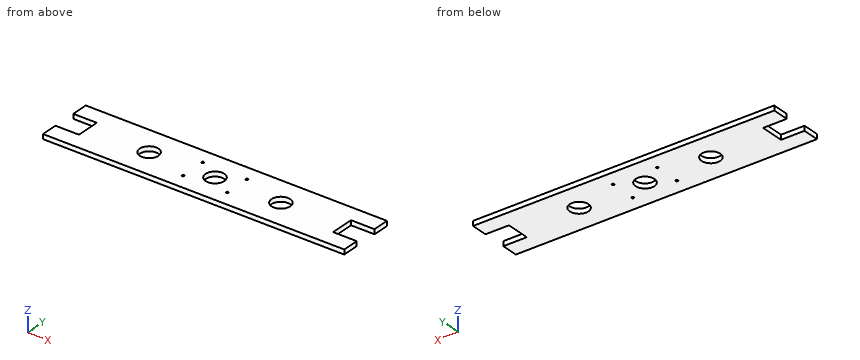
from build123d import *

# Parameters (mm, degrees)
F0_R     = 3.175
F0_R_2   = 25.4
F1_DEPTH = 12.7


with BuildPart() as f1:
    # F0 (on Top) → F1 (new body)
    with BuildSketch(Plane.XY):
        Polygon((406.4, 76.2), (-406.4, 76.2), (-406.4, 31.75), (-342.9, 31.75), (-342.9, -31.75), (-406.4, -31.75), (-406.4, -76.2), (406.4, -76.2), (406.4, -31.75), (342.9, -31.75), (342.9, 31.75), (406.4, 31.75), align=None)
        with Locations((-59.5122, -34.925)):
            Circle(F0_R, mode=Mode.SUBTRACT)
        with Locations((59.5122, -34.925)):
            Circle(F0_R, mode=Mode.SUBTRACT)
        with Locations((-177.8, 0)):
            Circle(F0_R_2, mode=Mode.SUBTRACT)
        Circle(F0_R_2, mode=Mode.SUBTRACT)
        with Locations((-59.5122, 34.925)):
            Circle(F0_R, mode=Mode.SUBTRACT)
        with Locations((177.8, 0)):
            Circle(F0_R_2, mode=Mode.SUBTRACT)
        with Locations((59.5122, 34.925)):
            Circle(F0_R, mode=Mode.SUBTRACT)
    extrude(amount=F1_DEPTH)


solid = f1.part
Check sheet for the modelled part. Datum: model origin and axes. Units: mm. Round coordinates to 2 decimals unless told otherwise and drop trailing zeros. Loops run counter-clockwise (first coordinate to the right, second up) from the corner with the lowest first, then second, coordinate; pieces in that order, holes last. Notation, with made-up numbers: M -21,33.25 L 21,33.25 A22 cw 21,59.25 Z; hole C 1,75 d9. An arc over 180 degrees is marked long. One line per question, with ' | ' between items. Start each with the question number.
Item 1: Section check A-A (y = 0). Record the boundary of the cut face in (x, z).
Item 2: Gauge pin test, flat ends, axial feed: pin 1 Ø7.5 at (x, y) = (-59.51, 34.92) entering from -Z; pin 2 Ø3 at (y, z) = (-26.5, 5.5) entering from +X; pin 3 Ø3 at (y, z) = (26.5, 2) entering from -X. Record the tip position at first contact, or that the pin passes through.
Item 3: Scan lines: probe 1 along X at (y, z) = (23.5, 4.5); probe 2 along Y at (x, z) = (-372, 5.75); probe 3 along X at (y, z) = (10.5, 8.25). Record each from-to range of solid material in increasing order.
Item 4: Section check C-C (z = 10.5). Record the boundary of the cut face in (x, y) (3 decimals).
Item 5: Section check B-B (x = 177.8). Record the boundary of the cut face in (y, z), and give its area (3 significant figures).
Worked out:
1) outline: M -342.9,0 L -203.2,0 L -203.2,12.7 L -342.9,12.7 Z; M -152.4,0 L -25.4,0 L -25.4,12.7 L -152.4,12.7 Z; M 25.4,0 L 152.4,0 L 152.4,12.7 L 25.4,12.7 Z; M 203.2,0 L 342.9,0 L 342.9,12.7 L 203.2,12.7 Z
2) pin 1: z = 0 | pin 2: x = 342.9 | pin 3: x = -342.9
3) probe 1: -342.9 to -187.44, -168.16 to -9.64, 9.64 to 168.16, 187.44 to 342.9 | probe 2: -76.2 to -31.75, 31.75 to 76.2 | probe 3: -342.9 to -200.93, -154.67 to -23.13, 23.13 to 154.67, 200.93 to 342.9
4) outline: M -406.4,-76.2 L 406.4,-76.2 L 406.4,-31.75 L 342.9,-31.75 L 342.9,31.75 L 406.4,31.75 L 406.4,76.2 L -406.4,76.2 L -406.4,31.75 L -342.9,31.75 L -342.9,-31.75 L -406.4,-31.75 Z; hole C -177.8,0 d50.8; hole C -59.512,-34.925 d6.35; hole C -59.512,34.925 d6.35; hole C 0,0 d50.8; hole C 59.512,-34.925 d6.35; hole C 59.512,34.925 d6.35; hole C 177.8,0 d50.8
5) outline: M -76.2,0 L -25.4,0 L -25.4,12.7 L -76.2,12.7 Z; M 25.4,0 L 76.2,0 L 76.2,12.7 L 25.4,12.7 Z | area: 1,290 mm^2
